Source: three-view drawing plus pictorial views. Frame: mm from the lowest corner of the part. A direction names the side the tool comes from. Give positions to 0.01 mm unless a question says otherwise; leave off trailing zeros. Loops run counter-clockwise (first coordinate to the right, second up) from the corner with the lowest first, then second, coordinate; pieces in that order, holes last. Notation, with made-up numbers: (2.25, 69.25) - (9.25, 69.25) arc R24 cw to (9.25, 106.25) - close; hole circle Ø9 at (5, 71.5). An arc over 180 degrees is marked (long way). Answer as a JSON object with one key per item and string values.
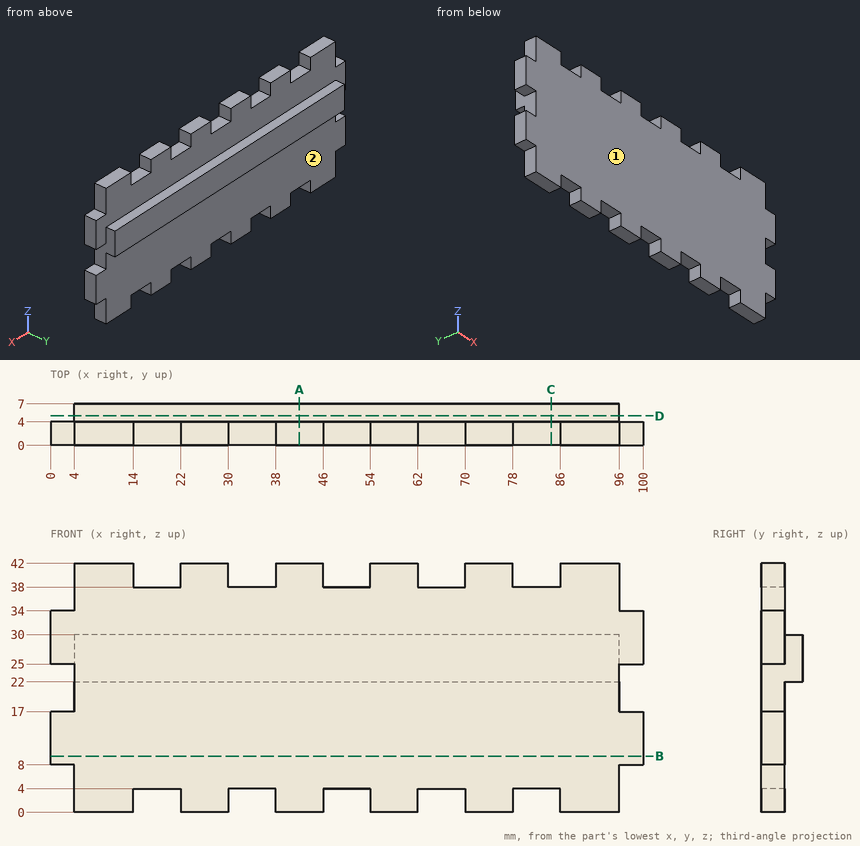
Item 1: Cut plane D-D (y = 5). Return loops of the section in (x, z), then the cut area to 3 significant figures.
Geometry check:
{"outline": "(4, 22) - (96, 22) - (96, 30) - (4, 30) - close", "area": "736 mm2"}
Item 2: Access query for the marked faces 1 and 2. Directions: +Z, -Z, +X, -X, +Y, -Y. A direction counts if a zero-diameter tool reaches every point of the face in a straight line with its end or side. Return the directions, or none.
Geometry check:
{"face 1": "+Z, -Z, +X, -X, -Y", "face 2": "-Z, +X, -X, +Y"}
Item 3: Cut plane A-A (x = 42). Return loops of the section in (y, z), then the cut area to 3 significant figures.
Geometry check:
{"outline": "(0, 0) - (4, 0) - (4, 22) - (7, 22) - (7, 30) - (4, 30) - (4, 42) - (0, 42) - close", "area": "192 mm2"}
Item 4: Contact query for flat-ended pins moving along their axis: P1, Ø2, axis at y = 2, z = 2.5, coming from the +X side; P2, Ø1.2, axis at x = 32.5, y = 2, coming from the -Z side; P3, Ø1.2, axis at y = 2, z = 39.5, coming from the -X side. Output: stop coordinate, or through.
Geometry check:
{"P1": "stops at x = 96", "P2": "stops at z = 4", "P3": "stops at x = 4"}
Item 5: Material intervals for line 1 (X direction, y = 2.5, z = 38.5); line 2 (Y direction, x = 35, z = 13); line 3 (Z direction, x = 9, y = 5.5), sorted ascending. Write a range as [from, to].
Geometry check:
{"line 1": "x = [4, 14], [22, 30], [38, 46], [54, 62], [70, 78], [86, 96]", "line 2": "y = [0, 4]", "line 3": "z = [22, 30]"}
Item 6: Cut plane C-C (x = 84.5). Return loops of the section in (y, z), then the cut area to 3 significant figures.
Geometry check:
{"outline": "(0, 4) - (4, 4) - (4, 22) - (7, 22) - (7, 30) - (4, 30) - (4, 38) - (0, 38) - close", "area": "160 mm2"}
Item 7: Cut plane B-B (z = 9.5). Return loops of the section in (x, y), then the cut area to 3 significant figures.
Geometry check:
{"outline": "(0, 0) - (100, 0) - (100, 4) - (0, 4) - close", "area": "400 mm2"}
